Design review of the part built by this model. Coordinates are the model's own, in mm. Face numbers are marked on the shaded views. A direction names the side the tool comes from. Coordinates: 2 decimals unless noted, no trailing zeros. Write each loop counter-clockwise with the first axis right and the second up, starting at its lowest first coordinate (ties: lowest second). Pieces come first, ordered by that corner, then holes.
Q1. For the marked faces 4 and 5, list the 3-axis set-ups (+Z, -Z, +X, -X, +Y, -Y) from which the entire face can be reached by the end or side of a thin tool; tool diameter is ignored.
Q2. Take a section at B-B, the plane y = 16.25. Write out the cut boundary in (x, z).
Q3. For L1, parallel to Y at x = -1, z = 1.25; L2, parallel to Y at x = 2.5, z = 0.75; L3, parallel to Z at x = 0, y = 5.25, list the stretches that pass through material, from the lowest coordinate up.
Q4. The part is to be moulded in two halves that separate along Y. For the marked faces 1, 2 and 3, say which applies: released by +Y, released by -Y, zero draft, split by the parting line, or undercut.
Q5. Take a section at A-A, the plane y = 6.5. Write out the cut boundary in (x, z), plus the area to 3 significant figures.
Q6. For pin 1 Ø1 at (x, z) = (-0.5, -1) entering from +Y; pin 2 Ø2 at (x, z) = (0, -1.5) entering from +Y; pin 3 Ø1 at (y, z) = (12, 1.5) entering from +X, all flat-tipped, find the tip position at first contact; note any pin that passes through.
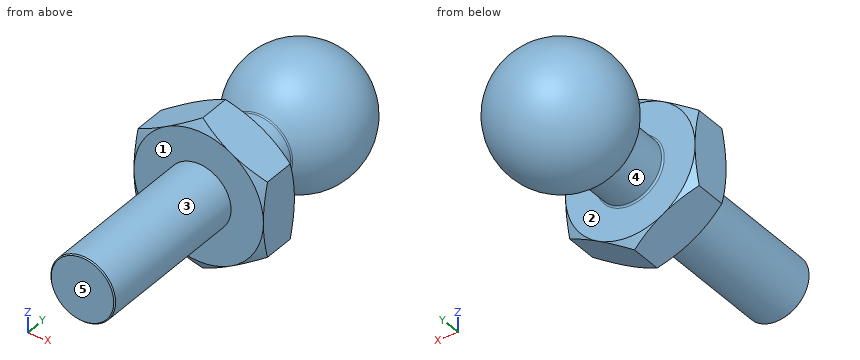
from build123d import *

# Parameters (mm, degrees)
CHAMFER1_SIZE       = 0.05
SKETCH4_R           = 1.5
BOSS_EXTRUDE2_DEPTH = 2
SKETCH5_OUTSIDE_W   = 18.79
SKETCH5_OUTSIDE_H   = 19.718
SKETCH5_OUTSIDE_R   = 3
CUT_EXTRUDE1_DEPTH  = 2
CUT_EXTRUDE1_TAPER  = 60
SKETCH6_OUTSIDE_W   = 18.79
SKETCH6_OUTSIDE_H   = 19.718
SKETCH6_OUTSIDE_R   = 3
CUT_EXTRUDE2_DEPTH  = 2
CUT_EXTRUDE2_TAPER  = 60
FILLET1_R           = 0.075


with BuildPart() as part:
    # Sketch1 → Revolve2 (revolve)
    with BuildSketch(Plane.XY):
        with BuildLine():
            Line((0, 0), (0, 11))
            Line((0, 11), (0, 17))
            ThreePointArc((0, 17), (2.897777479, 14.776457135), (1.5, 11.401923789))
            Line((1.5, 11.401923789), (1.5, 0))
            Line((1.5, 0), (0, 0))
        make_face()
    revolve(axis=Axis((0, 0, 0), (0, 1, 0)))

    # Chamfer1
    chamfer1_edges = [part.edges().sort_by_distance(p)[0] for p in [
        (-1.5, 0, 0),
    ]]
    chamfer(chamfer1_edges, length=CHAMFER1_SIZE)

    # Sketch4 → Boss-Extrude2 (add)
    with BuildSketch(Plane(origin=(0, 7.5, 0), x_dir=(1, 0, 0), z_dir=(0, 1, 0))):
        Polygon((0, -3.464101615), (3, -1.732050808), (3, 1.732050808), (0, 3.464101615), (-3, 1.732050808), (-3, -1.732050808), align=None)
        Circle(SKETCH4_R, mode=Mode.SUBTRACT)
    extrude(amount=BOSS_EXTRUDE2_DEPTH)

    # Sketch5 outside → Cut-Extrude1 (cut)
    with BuildSketch(Plane.XZ.offset(-7.5)):
        Rectangle(SKETCH5_OUTSIDE_W, SKETCH5_OUTSIDE_H)
        Circle(SKETCH5_OUTSIDE_R, mode=Mode.SUBTRACT)
    extrude(amount=-CUT_EXTRUDE1_DEPTH, taper=CUT_EXTRUDE1_TAPER, mode=Mode.SUBTRACT)

    # Sketch6 outside → Cut-Extrude2 (cut)
    with BuildSketch(Plane(origin=(0, 9.5, 0), x_dir=(1, 0, 0), z_dir=(0, 1, 0))):
        Rectangle(SKETCH6_OUTSIDE_W, SKETCH6_OUTSIDE_H)
        Circle(SKETCH6_OUTSIDE_R, mode=Mode.SUBTRACT)
    extrude(amount=-CUT_EXTRUDE2_DEPTH, taper=CUT_EXTRUDE2_TAPER, mode=Mode.SUBTRACT)

    # Fillet1
    fillet1_edges = [part.edges().sort_by_distance(p)[0] for p in [
        (-1.5, 9.5, 0),
        (-1.5, 11.401923789, 0),
    ]]
    fillet(fillet1_edges, radius=FILLET1_R)


solid = part.part
Responses:
1. face 4: none
1. face 5: +Z, -Z, +X, -X, -Y
2. outline: circle Ø3.97 at (0, 0)
3. L1: y = 7.5 to 9.5, 11.46 to 16.54
3. L2: y = 7.5 to 9.5, 12.52 to 15.48
3. L3: z = -1.5 to 1.5
4. face 1: released by -Y
4. face 2: undercut
4. face 3: zero draft
5. outline: circle Ø3 at (0, 0)
5. area: 7.07 mm2
6. pin 1: stops at y = 16.94
6. pin 2: stops at y = 16.96
6. pin 3: stops at x = 2.24
